Check sheet for the modelled part. Datum: model origin and axes. Units: mm. Face numbers are marked on the shaded views. A direction names the side the tool comes from. Coordinates: 2 decimals unless noted, no trailing zeros. Loops run counter-clockwise (first coordinate to the right, second up) from the corner with the lowest first, then second, coordinate; pieces in that order, holes last. Notation, with made-up numbers: (62.25, 55.25) -> (76.25, 55.25) arc R21 ccw to (76.25, 77.25) -> close; hole circle Ø8 at (42.5, 4). An arc over 180 degrees is marked (long way). Use one line per item in the form item = value.
Autodesk Inventor part; units mm, degrees
ref_plane "hh_XY" through (0, 4.7625, 0) normal (0, 0, 1) x (1, 0, 0)
ref_plane "hh_YZ" through (0, 4.7625, 0) normal (1, 0, 0) x (0, 1, 0)
ref_plane "hh_ZX" through (0, 4.7625, 0) normal (0, 1, 0) x (0, 0, 1)
sketch "Sketch_1" plane through (0, 0, 0) normal (0, 0, 1) x (1, 0, 0)
  line L0 (7.9248, 0) -> (0, 0)
  line L1 (0, 0) -> (0, 4.1326)
  line L2 (0, 4.1326) -> (0.6299, 4.7625)
  line L3 (0.6299, 4.7625) -> (7.9248, 4.7625)
  line L4 (7.9248, 4.7625) -> (7.9248, 0)
  line L5 (7.9248, 0) -> (0, 0)
revolve "Revolution1" add sketch "Sketch_1" angle 360 about axis through (7.9248, 0, 0) along (1, 0, 0)
thread "Thread1"
sketch "Sketch_3" plane through (0, 0, 0) normal (0, 0, 1) x (1, 0, 0)
  line L0 (21.463, 0) -> (7.9248, 0)
  line L1 (7.9248, 0) -> (7.9248, 6.9215)
  line L2 (7.9248, 6.9215) -> (8.6868, 7.6835)
  line L3 (8.6868, 7.6835) -> (15.1003, 7.6835)
  line L4 (15.1003, 7.6835) -> (15.8623, 6.9215)
  line L5 (15.8623, 6.9215) -> (15.8623, 3.5243)
  line L6 (15.8623, 3.5243) -> (17.9959, 3.5243)
  line L7 (17.9959, 3.5243) -> (18.5547, 4.0831)
  line L8 (18.5547, 4.0831) -> (20.955, 4.0831)
  line L9 (20.955, 4.0831) -> (21.463, 3.575)
  line L10 (21.463, 3.575) -> (21.463, 0)
  line L11 (21.463, 0) -> (7.9248, 0)
revolve "Revolution2" add sketch "Sketch_3" angle 360 about axis through (21.463, 0, 0) along (1, 0, 0)
sketch "Sketch_17" plane through (0, 0, 0) normal (0, 0, 1) x (1, 0, 0)
  line L0 (17.4371, 0) -> (15.8623, 0)
  line L1 (15.8623, 0) -> (15.8623, 4.5593)
  line L2 (15.8623, 4.5593) -> (17.4371, 4.5593)
  line L3 (17.4371, 4.5593) -> (17.4371, 0)
  line L4 (17.4371, 0) -> (15.8623, 0)
revolve "Revolution3" add sketch "Sketch_17" angle 360 about axis through (17.4371, 0, 0) along (1, 0, 0)
sketch "Sketch4" plane through (0, 0, 0) normal (-1, 0, 0) x (0, 0, 1)
  point P0 (0, 0)
hole "Hole1" at (0, 0, 0) direction (1, 0, 0) diameter 3.2512 depth 21.463 countersink diameter 4.0132 countersink angle 90
sketch "Sketch_16" plane through (0, 0, 0) normal (1, 0, 0) x (0, 1, 0)
  line L0 (-12.7, 12.7) -> (-12.7, -12.7)
  line L1 (-12.7, -12.7) -> (12.7, -12.7)
  line L2 (12.7, -12.7) -> (12.7, 12.7)
  line L3 (12.7, 12.7) -> (-12.7, 12.7)
  line L4 (-6.35, 6.35) -> (-6.35, -6.35)
  line L5 (-6.35, -6.35) -> (6.35, -6.35)
  line L6 (6.35, -6.35) -> (6.35, 6.35)
  line L7 (6.35, 6.35) -> (-6.35, 6.35)
extrude "Extrusion1" cut sketch "Sketch_16" along normal blind 21.463
sketch "Sketch6" plane through (8.6868, -4.3259, 6.35) normal (0, 0, 1) x (1, 0, 0)
  point P0 (3.2512, 4.3259)
hole "Hole2" at (11.938, 0, 6.35) direction (0, 0, -1) diameter 3.9624 depth 6.35 countersink diameter 4.826 countersink angle 90
sketch "Sketch_47" plane through (0, 0, 0) normal (0, 0, 1) x (1, 0, 0)
  line L0 (17.9959, 0) -> (17.4371, 0)
  line L1 (17.4371, 4.0431) -> (17.4371, 3.2702)
  line L2 (17.4371, 3.2702) -> (17.9959, 3.2702)
  line L3 (17.9959, 3.2702) -> (17.9959, 3.5243)
  line L4 (17.9959, 3.5243) -> (17.7165, 3.5243)
  line L5 (17.7165, 3.5243) -> (17.5509, 3.6899)
  arc A0 (17.5509, 3.8695) -> (17.5509, 3.6899) centre (17.6407, 3.7797) ccw
  line L6 (17.5509, 3.8695) -> (18.1565, 4.4751)
  line L7 (18.1565, 4.4751) -> (18.1565, 4.5593)
  line L8 (18.1565, 4.5593) -> (17.9533, 4.5593)
  line L9 (17.9533, 4.5593) -> (17.4371, 4.0431)
revolve "Revolution4" add sketch "Sketch_47" angle 360 about axis through (17.9959, 0, 0) along (1, 0, 0)
ref_plane "hh_XY" through (0, 4.7625, 0) normal (0, 0, 1) x (1, 0, 0)
ref_plane "hh_YZ" through (0, 4.7625, 0) normal (1, 0, 0) x (0, 1, 0)
ref_plane "hh_ZX" through (0, 4.7625, 0) normal (0, 1, 0) x (0, 0, 1)
ref_plane "port_XY" through (11.938, 0, 0) normal (0, 0, 1) x (1, 0, 0)
ref_plane "port_YZ" through (11.938, 0, 0) normal (1, 0, 0) x (0, 1, 0)
ref_plane "port_ZX" through (11.938, 0, 0) normal (0, 1, 0) x (0, 0, 1)
ref_plane "rod_guide_XY" through (0, 0, 0) normal (1, 0, 0) x (0, 0, -1)
ref_plane "rod_guide_YZ" through (0, 0, 0) normal (0, 0, -1) x (0, 1, 0)
ref_plane "rod_guide_ZX" through (0, 0, 0) normal (0, 1, 0) x (1, 0, 0)
ref_plane "sq1_XY" through (0, 0, 6.35) normal (1, 0, 0) x (0, 0, -1)
ref_plane "sq1_YZ" through (0, 0, 6.35) normal (0, 0, -1) x (0, 1, 0)
ref_plane "sq1_ZX" through (0, 0, 6.35) normal (0, 1, 0) x (1, 0, 0)
ref_plane "sq2_XY" through (0, 0, -6.35) normal (1, 0, 0) x (0, 0, -1)
ref_plane "sq2_YZ" through (0, 0, -6.35) normal (0, 0, -1) x (0, 1, 0)
ref_plane "sq2_ZX" through (0, 0, -6.35) normal (0, 1, 0) x (1, 0, 0)
ref_plane "t1_XY" through (7.9248, 0, 0) normal (1, 0, 0) x (0, 0, -1)
ref_plane "t1_YZ" through (7.9248, 0, 0) normal (0, 0, -1) x (0, 1, 0)
ref_plane "t1_ZX" through (7.9248, 0, 0) normal (0, 1, 0) x (1, 0, 0)
ref_plane "t111_XY" through (7.9248, 0, 0) normal (1, 0, 0) x (0, 0, -1)
ref_plane "t111_YZ" through (7.9248, 0, 0) normal (0, 0, -1) x (0, 1, 0)
ref_plane "t111_ZX" through (7.9248, 0, 0) normal (0, 1, 0) x (1, 0, 0)
ref_plane "to_foot_bracket_XY" through (7.9248, 0, 0) normal (1, 0, 0) x (0, 0, -1)
ref_plane "to_foot_bracket_YZ" through (7.9248, 0, 0) normal (0, 0, -1) x (0, 1, 0)
ref_plane "to_foot_bracket_ZX" through (7.9248, 0, 0) normal (0, 1, 0) x (1, 0, 0)
ref_plane "to_nut_XY" through (7.9248, 0, 0) normal (1, 0, 0) x (0, 0, -1)
ref_plane "to_nut_YZ" through (7.9248, 0, 0) normal (0, 0, -1) x (0, 1, 0)
ref_plane "to_nut_ZX" through (7.9248, 0, 0) normal (0, 1, 0) x (1, 0, 0)
ref_plane "to_rod_XY" through (-18.415, 0, 0) normal (1, 0, 0) x (0, 0, -1)
ref_plane "to_rod_YZ" through (-18.415, 0, 0) normal (0, 0, -1) x (0, 1, 0)
ref_plane "to_rod_ZX" through (-18.415, 0, 0) normal (0, 1, 0) x (1, 0, 0)
ref_plane "to_screw_XY" through (11.938, 0, 0) normal (0, 1, 0) x (1, 0, 0)
ref_plane "to_screw_YZ" through (11.938, 0, 0) normal (1, 0, 0) x (0, 0, -1)
ref_plane "to_screw_ZX" through (11.938, 0, 0) normal (0, 0, -1) x (0, 1, 0)
ref_plane "to_trunnion_brackets_XY" through (0, 0, 0) normal (0, 1, 0) x (1, 0, 0)
ref_plane "to_trunnion_brackets_YZ" through (0, 0, 0) normal (1, 0, 0) x (0, 0, -1)
ref_plane "to_trunnion_brackets_ZX" through (0, 0, 0) normal (0, 0, -1) x (0, 1, 0)
ref_plane "to_trunnion_brackets1_XY" through (0, 6.35, 0) normal (0, 1, 0) x (1, 0, 0)
ref_plane "to_trunnion_brackets1_YZ" through (0, 6.35, 0) normal (1, 0, 0) x (0, 0, -1)
ref_plane "to_trunnion_brackets1_ZX" through (0, 6.35, 0) normal (0, 0, -1) x (0, 1, 0)
ref_plane "to_trunnion_brackets2_XY" through (0, -6.35, 0) normal (0, 1, 0) x (1, 0, 0)
ref_plane "to_trunnion_brackets2_YZ" through (0, -6.35, 0) normal (1, 0, 0) x (0, 0, -1)
ref_plane "to_trunnion_brackets2_ZX" through (0, -6.35, 0) normal (0, 0, -1) x (0, 1, 0)
ref_plane "to_tube_XY" through (17.9959, 0, 0) normal (1, 0, 0) x (0, 0, -1)
ref_plane "to_tube_YZ" through (17.9959, 0, 0) normal (0, 0, -1) x (0, 1, 0)
ref_plane "to_tube_ZX" through (17.9959, 0, 0) normal (0, 1, 0) x (1, 0, 0)
properties part number "007R000-0.725_rod_guide"
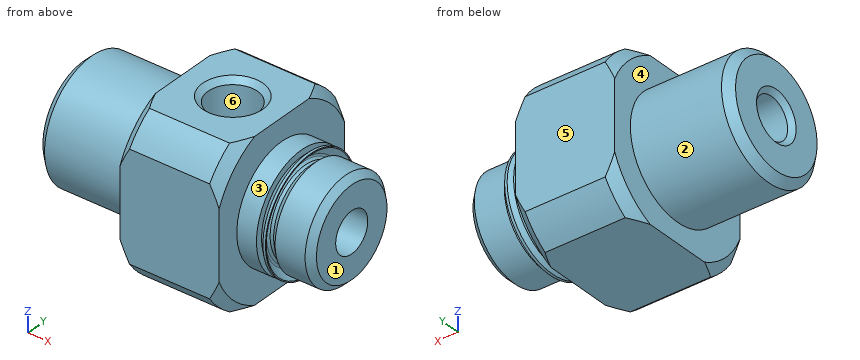
(1) Scan lines: line 1 along Y through (x, z) = (10.25, 0); line 2 along X through (y, z) = (0, 3.2); line 3 along Z through (x, y) = (12, 0). Record each from-to range of solid material in increasing order.
Established:
line_1 = -6.35 to -1.63, 1.63 to 6.35
line_2 = 0 to 9.96, 13.92 to 21.46
line_3 = -6.35 to -1.63
(2) Mould release check, pull along Y, two halves, no side actions. Record for the marked faces 4, 5 and 6: +Y half, -Y half, draft (parallel to the pull), parting line (faces both ways), or undercut.
Established:
face_4 = draft
face_5 = +Y half
face_6 = undercut
(3) Tool access check on the marked faces 1, 2 and 3. Record the directions out of +Z, -Z, +X, -X, +Y, -Y that give a thin tool (end or side, any length) a straight path to the whole face; none if there is none.
Established:
face_1 = +Z, -Z, +X, +Y, -Y
face_2 = -X
face_3 = +X
(4) Section check A-A, the plane x = 9. Record the boundary of the cut face in (y, z), plus the area to 3 significant figures.
Established:
outline = (-6.35, -4.33) arc R7.68 ccw to (-4.33, -6.35) -> (4.33, -6.35) arc R7.68 ccw to (6.35, -4.33) -> (6.35, 4.33) arc R7.68 ccw to (4.33, 6.35) -> (-4.33, 6.35) arc R7.68 ccw to (-6.35, 4.33) -> close; hole circle Ø3.25 at (0, 0)
area = 146 mm²
(5) Section check B-B, the plane y = 0. Give the number of separate pieces and of enclosed holes in the cut face, plus the area to 3 significant figures.
Established:
separate_pieces = 3
enclosed_holes = 0
area = 134 mm²
(6) Go/stop test with flat-tipped pins: P1, Ø6, axis at x = 14, y = 4.5, coming from the +Z side; P2, Ø1.5, axis at x = 17.5, z = 3, coming from the +Y side; P3, Ø1, axis at x = 19.5, y = -1, coming from the -Z side; P4, Ø1, axis at x = 4.5, y = 1, coming from the -Z side. Record where each tip stops, or that it passes through.
Established:
P1 = 6.35
P2 = 3.96
P3 = -4.05
P4 = -4.74
(7) Section check C-C, the plane x = 16.5. Record the boundary of the cut face in (y, z).
Established:
outline = circle Ø9.12 at (0, 0); hole circle Ø3.25 at (0, 0)
(8) Section check D-D, the plane x = 4. Record the boundary of the cut face in (y, z) (1 decimal).
Established:
outline = circle Ø9.5 at (0, 0); hole circle Ø3.3 at (0, 0)
